```python
from build123d import *

# Parameters (mm, degrees)
SKETCH2_W            = 115.8875
SKETCH2_H            = 122.2375
BOSS_EXTRUDE4_DEPTH  = 1.5875
M4_CLEARANCE_HOLE1_D = 4.5
FILLET1_R            = 19.05
FILLET2_R            = 6.35
FILLET3_R            = 3.175


with BuildPart() as part:
    # Sketch2 → Boss-Extrude4 (new body)
    with BuildSketch(Plane(origin=(0, 0, 0), x_dir=(1, 0, 0), z_dir=(0, 1, 0))):
        with Locations((-95.437748261, 114.593960112)):
            Rectangle(SKETCH2_W, SKETCH2_H)
        Polygon((-133.696498261, 160.155210112), (-60.951469128, 160.155210112), (-133.696498261, 83.253322171), align=None, mode=Mode.SUBTRACT)
        Polygon((-52.416498261, 150.697098052), (-52.416498261, 73.795210112), (-125.161527393, 73.795210112), align=None, mode=Mode.SUBTRACT)
    extrude(amount=BOSS_EXTRUDE4_DEPTH)

    # M4 Clearance Hole1 (through all)
    with Locations(Plane(origin=(0, 1.5875, 0), x_dir=(1, 0, 0), z_dir=(0, 1, 0))):
        with Locations((-93.056498261, 65.065510112), (-137.14786851, 69.38383987), (-141.466198251, 116.975210121), (-137.147868492, 164.56658037), (-93.056498242, 168.884910112), (-48.965127993, 164.566580353), (-44.646798251, 116.975210102), (-48.965128011, 69.383839853)):
            Hole(M4_CLEARANCE_HOLE1_D / 2)

    # Fillet1
    fillet1_edges = [part.edges().sort_by_distance(p)[0] for p in [
        (-37.493998261, 0.79375, -175.712710112),
    ]]
    fillet(fillet1_edges, radius=FILLET1_R)

    # Fillet2
    fillet2_edges = [part.edges().sort_by_distance(p)[0] for p in [
        (-133.696498261, 0.79375, -160.155210112),
        (-52.416498261, 0.79375, -73.795210112),
    ]]
    fillet(fillet2_edges, radius=FILLET2_R)

    # Fillet3
    fillet3_edges = [part.edges().sort_by_distance(p)[0] for p in [
        (-133.696498261, 0.79375, -83.253322171),
        (-60.951469128, 0.79375, -160.155210112),
        (-125.161527393, 0.79375, -73.795210112),
        (-52.416498261, 0.79375, -150.697098052),
    ]]
    fillet(fillet3_edges, radius=FILLET3_R)


solid = part.part
```
Build history of the part. All positions in model axes, mm. A direction names the side the tool comes from. Round coordinates to 2 decimals unless told otherwise and drop trailing zeros. Order: outer loops, then holes, each group sorted by start corner. A loop starts at its lowest first (then second) coordinate and runs counter-clockwise, first axis right, second up. Notation, with made-up numbers: (89, 65.25) -> (114, 65.25) arc R18 cw to (114, 95.25) -> close; hole circle Ø3 at (71, 48.5). An arc over 180 degrees is marked (long way). Answer in a Markdown table with one row per item.
1) Band-saw the part on C-C on z = -121.5. Give the cut face in (x, y), and give its area (3 significant figures).
Values:
| item | result |
|---|---|
| outline | (-153.38, 0) -> (-133.7, 0) -> (-133.7, 1.59) -> (-153.38, 1.59) -> close; (-97.52, 0) -> (-80.04, 0) -> (-80.04, 1.59) -> (-97.52, 1.59) -> close; (-52.42, 0) -> (-37.49, 0) -> (-37.49, 1.59) -> (-52.42, 1.59) -> close |
| area | 82.7 mm2 |
2) Wall check: L1, parallel to Z at x = -114.5, y = 0.5; L2, parallel to Z at x = -79, y = 1.4; L3, parallel to X at y = 0.3, z = -131. Give the ranges that are in metal, low to high.
Values:
| item | result |
|---|---|
| L1 | -175.71 to -160.16, -103.55 to -85.07, -73.8 to -53.48 |
| L2 | -175.71 to -160.16, -141.08 to -122.59, -73.8 to -53.48 |
| L3 | -153.38 to -133.7, -88.53 to -71.05, -52.42 to -37.49 |
3) Pin check, flat tip, straight feed: P1, Ø2.5, axis at x = -44.65, z = -116.98, coming from the -Y side. Stop position of the tip, or through.
Values:
| item | result |
|---|---|
| P1 | through |
4) Which spindle directions (+Z, -Z, +X, -X, +Y, -Y) get a long thin tool onto all of the face, cutting with end or side? Do faces 1 (the cylindrical face through (-54.326, 0.805, -75.606)), 2 (the flat face through (-96, 1.588, -115)). Say none if no direction does.
Values:
| item | result |
|---|---|
| face 1 | +Y, -Y |
| face 2 | +Z, -Z, +X, -X, +Y |
5) Band-saw the part on D-D on z = -150. Give the cut face in (x, y).
Values:
| item | result |
|---|---|
| outline | (-153.38, 0) -> (-133.7, 0) -> (-133.7, 1.59) -> (-153.38, 1.59) -> close; (-70.56, 0) -> (-37.49, 0) -> (-37.49, 1.59) -> (-70.56, 1.59) -> close |
6) Band-saw the part on A-A on y = 0.6. Give the number of separate pieces and of enclosed holes in the cut face, and give its area (3 significant figures).
Values:
| item | result |
|---|---|
| separate pieces | 1 |
| enclosed holes | 10 |
| area | 8,430 mm2 |
7) Band-saw the part on B-B on x = -72. Give the cut face in (y, z).
Values:
| item | result |
|---|---|
| outline | (0, -175.71) -> (1.59, -175.71) -> (1.59, -160.16) -> (0, -160.16) -> close; (0, -148.48) -> (1.59, -148.48) -> (1.59, -129.99) -> (0, -129.99) -> close; (0, -73.8) -> (1.59, -73.8) -> (1.59, -53.48) -> (0, -53.48) -> close |
8) Mould opens along X. For faces 3 (the cylindrical face through (-120.683, 0.805, -75.667)), 4 (the cylindrical face through (-43.22, 0.8, -170.28)), 5 (the flat face through (-96, 0, -115)) say: released by +X, released by -X, zero draft, split by the parting line, or undercut.
Values:
| item | result |
|---|---|
| face 3 | undercut |
| face 4 | released by +X |
| face 5 | zero draft |
